```python
from build123d import *

# Parameters (mm, degrees)
EXTRUDE_1_DEPTH      = 100
SKETCH_2_R           = 40
CUT_EXTRUDE_1_DEPTH  = 90
SKETCH_9_W           = 96.5
SKETCH_9_H           = 96.5
CUT_EXTRUDE_3_DEPTH  = 100
SKETCH_15_R          = 4
EXTRUDE_4_DEPTH      = 5
SKETCH_16_R          = 29.5
CUT_EXTRUDE_5_DEPTH  = 5
SKETCH_19_W          = 96.5
SKETCH_19_H          = 96.5
CUT_EXTRUDE_8_DEPTH  = 99
SKETCH_20_R          = 2
SKETCH_20_R_2        = 4
CUT_EXTRUDE_9_DEPTH  = 1.75
SKETCH_23_W          = 92
SKETCH_23_H          = 92
EXTRUDE_5_DEPTH      = 57.3
SKETCH_24_R          = 1.75
SKETCH_24_R_2        = 4
CUT_EXTRUDE_10_DEPTH = 3
CUT_EXTRUDE_START    = -5
SKETCH_27_W          = 92
SKETCH_27_H          = 92
CUT_EXTRUDE_12_DEPTH = 50
FILLET_2_R           = 3
FILLET_6_R           = 15


with BuildPart() as part:
    # 草图1 → 凸台-拉伸1 (new body)
    with BuildSketch(Plane(origin=(0, 0, 0), x_dir=(1, 0, 0), z_dir=(0, 1, 0))):
        Polygon((-50, 50), (-50, 150), (50, 150), (150, 150), (150, 50), (50, 50), (50, -50), (-50, -50), align=None)
    extrude(amount=EXTRUDE_1_DEPTH)

    # 草图2 → 切除-拉伸1 (cut)
    with BuildSketch(Plane(origin=(0, 100, 0), x_dir=(1, 0, 0), z_dir=(0, 1, 0))):
        with Locations(Location((0, 0, 0), (0, 0, 270))):
            Circle(SKETCH_2_R)
    extrude(amount=-CUT_EXTRUDE_1_DEPTH, mode=Mode.SUBTRACT)

    # 草图9 → 切除-拉伸3 (cut)
    with BuildSketch(Plane.ZY.offset(50)):
        with Locations((0, 50)):
            Rectangle(SKETCH_9_W, SKETCH_9_H)
    extrude(amount=-CUT_EXTRUDE_3_DEPTH, mode=Mode.SUBTRACT)

    # 草图15 → 凸台-拉伸4 (add)
    with BuildSketch(Plane(origin=(0, 0, -150), x_dir=(-1, 0, 0), z_dir=(0, 0, -1))):
        with Locations(Location((-89.023351099, 21, 0), (0, 0, 180))):
            Circle(SKETCH_15_R)
        with Locations(Location((-89.023351099, 79, 0), (0, 0, 180))):
            Circle(SKETCH_15_R)
    extrude(amount=EXTRUDE_4_DEPTH)

    # 草图16 → 切除-拉伸5 (cut)
    with BuildSketch(Plane.XZ):
        with Locations((100, -100)):
            Circle(SKETCH_16_R)
    extrude(amount=-CUT_EXTRUDE_5_DEPTH, mode=Mode.SUBTRACT)

    # 草图19 → 切除-拉伸8 (cut)
    with BuildSketch(Plane.XY.offset(-50)):
        with Locations((100, 50)):
            Rectangle(SKETCH_19_W, SKETCH_19_H)
    extrude(amount=-CUT_EXTRUDE_8_DEPTH, mode=Mode.SUBTRACT)

    # 草图20 → 切除-拉伸9 (cut)
    with BuildSketch(Plane(origin=(0, 1.75, 0), x_dir=(1, 0, 0), z_dir=(0, 1, 0))):
        with Locations(Location((17.25, 0, 0), (0, 0, 270))):
            Circle(SKETCH_20_R)
        with Locations(Location((8.625, -14.938938215, 0), (0, 0, 270))):
            Circle(SKETCH_20_R)
        with Locations(Location((-8.625, -14.938938215, 0), (0, 0, 270))):
            Circle(SKETCH_20_R)
        with Locations(Location((-17.25, 0, 0), (0, 0, 270))):
            Circle(SKETCH_20_R)
        with Locations(Location((-8.625, 14.938938215, 0), (0, 0, 270))):
            Circle(SKETCH_20_R)
        with Locations(Location((8.625, 14.938938215, 0), (0, 0, 270))):
            Circle(SKETCH_20_R)
        with Locations(Location((0, 0, 0), (0, 0, 270))):
            Circle(SKETCH_20_R_2)
    extrude(amount=-CUT_EXTRUDE_9_DEPTH, mode=Mode.SUBTRACT)

    # 草图23 → 凸台-拉伸5 (add)
    with BuildSketch(Plane(origin=(0, 100, 0), x_dir=(1, 0, 0), z_dir=(0, 1, 0))):
        with Locations((100, 100)):
            Rectangle(SKETCH_23_W, SKETCH_23_H)
    extrude(amount=-EXTRUDE_5_DEPTH)

    # 草图24 → 切除-拉伸10 (cut)
    with BuildSketch(Plane.XZ.offset(-42.7)):
        with Locations(Location((100, -57.5, 0), (0, 0, 270))):
            Circle(SKETCH_24_R)
        with Locations(Location((130.0520382, -69.9479618, 0), (0, 0, 270))):
            Circle(SKETCH_24_R)
        with Locations(Location((142.5, -100, 0), (0, 0, 270))):
            Circle(SKETCH_24_R)
        with Locations(Location((130.0520382, -130.0520382, 0), (0, 0, 270))):
            Circle(SKETCH_24_R)
        with Locations(Location((100, -142.5, 0), (0, 0, 270))):
            Circle(SKETCH_24_R)
        with Locations(Location((69.9479618, -130.0520382, 0), (0, 0, 270))):
            Circle(SKETCH_24_R)
        with Locations(Location((57.5, -100, 0), (0, 0, 270))):
            Circle(SKETCH_24_R)
        with Locations(Location((69.9479618, -69.9479618, 0), (0, 0, 270))):
            Circle(SKETCH_24_R)
        with Locations(Location((100, -100, 0), (0, 0, 270))):
            Circle(SKETCH_24_R_2)
    extrude(amount=-CUT_EXTRUDE_10_DEPTH, mode=Mode.SUBTRACT)

    # 草图27 → 切除-拉伸12 (cut)
    with BuildSketch(Plane(origin=(0, 100, 0), x_dir=(1, 0, 0), z_dir=(0, 1, 0)).offset(CUT_EXTRUDE_START)):
        with Locations((98.652941691, 99.180600888)):
            Rectangle(SKETCH_27_W, SKETCH_27_H)
    extrude(amount=-CUT_EXTRUDE_12_DEPTH, mode=Mode.SUBTRACT)

    # 圆角2
    # the kernel refuses this fillet: 3 mm, written as the material it takes off along each edge
    with BuildSketch(Plane(origin=(50, -7.5, 50), x_dir=(-1, 0, 0), z_dir=(0, 1, 0)), Plane(origin=(57.5, 0, 50), x_dir=(0, 0, -1), z_dir=(-1, 0, 0)), Plane(origin=(-50, -7.5, 50), x_dir=(0, 0, -1), z_dir=(0, 1, 0)), Plane(origin=(150, 0, -157.5), x_dir=(-1, 0, 0), z_dir=(0, 0, 1))) as fillet_2_piece_1:
        with BuildLine():
            CenterArc((FILLET_2_R, -FILLET_2_R), FILLET_2_R, 90, 90)
            Line((0, -FILLET_2_R), (0, 0))
            Line((0, 0), (FILLET_2_R, 0))
        make_face()
    extrude(amount=115, mode=Mode.SUBTRACT)
    with BuildSketch(Plane(origin=(57.5, 100, 50), x_dir=(0, 0, -1), z_dir=(-1, 0, 0)), Plane(origin=(150, 100, -157.5), x_dir=(-1, 0, 0), z_dir=(0, 0, 1)), Plane(origin=(150, -7.5, -50), x_dir=(0, 0, -1), z_dir=(0, 1, 0)), Plane(origin=(150, -7.5, -150), x_dir=(-1, 0, 0), z_dir=(0, 1, 0))) as fillet_2_piece_2:
        with BuildLine():
            CenterArc((FILLET_2_R, FILLET_2_R), FILLET_2_R, 180, 90)
            Line((0, FILLET_2_R), (0, 0))
            Line((0, 0), (FILLET_2_R, 0))
        make_face()
    extrude(amount=115, mode=Mode.SUBTRACT)

    # 圆角6
    fillet_6_edges = [part.edges().sort_by_distance(p)[0] for p in [
        (-50, 50, -150),
    ]]
    fillet(fillet_6_edges, radius=FILLET_6_R)


solid = part.part
```
Check sheet for the modelled part. Datum: model origin and axes. Units: mm. A direction names the side the tool comes from. Round coordinates to 2 decimals unless told otherwise and drop trailing zeros. Write each loop counter-clockwise with the first axis right and the second up, starting at its lowest first coordinate (ties: lowest second). Pieces come first, ordered by that corner, then holes. Notation, with made-up numbers: M 88,39.5 L 96,39.5 A14 cw 96,58.5 Z; hole C 45,83.25 d11. An arc over 180 degrees is marked long. Write item = value, one per line. Start each with the question number.
1. Gauge pin test, flat ends, axial feed: pin 1 (10 mm diameter, centred on x = -22, y = 17.5, fed in from -Z); pin 2 (6.5 mm diameter, centred on x = -8.62, z = -14.94, fed in from +Y); pin 3 (16.5 mm diameter, centred on x = 99, y = 64, fed in from +Z). Record the tip position at first contact, or that the pin passes through.
2. Section check C-C, the plane x = 81.5. Record the cut outline in (y, z), then the cut area to 3 significant figures.
3. Release check for a two-part mould opening along Z. For faces 5 (the flat face through (1, 49, 50)), 6 (the flat face through (-23, 98.25, -33)), 7 (the cylindrical face through (-39.05, 99.14, -8.67)), 8 (the flat face through (-50, 49, -86)) record: pulls with the +Z half, pulls with the -Z half, needs draft (parallel to the pull), parting line crosses it, or undercut.
4. Section check D-D, the plane z = -113.5. Record the cut outline in (x, y).
5. Section check A-A, the plane x = 44.5. Record the cut outline in (y, z).
6. Tool access check on faces 1 (the flat face through (53, 98.25, -99)), 2 (the flat face through (-1, 1.75, 10)), 3 (the flat face through (51.75, 49, -99)), 4 (the cylindrical face through (127.25, 0.86, -111.3)). Record the directions out of +Z, -Z, +X, -X, +Y, -Y that give a thin tool (end or side, any length) a straight path to the whole face; none if there is none.
7. Section check B-B, the plane z = -33.5. Record the cut outline in (x, y).
8. Scan lines: line 1 (Y direction, x = 132.5, z = -139); line 2 (X direction, y = 85, z = -110); line 3 (X direction, y = 43, z = -108). Record each from-to range of solid material in increasing order. Write a range as [from, to].
Results found:
q1.pin_1 = -150
q1.pin_2 = 1.75
q1.pin_3 = -145.18
q2.outline = M 0,-150 L 100,-150 L 100,-50 L 98.25,-50 L 98.25,-54 L 95,-54 L 95,-145.18 L 45,-145.18 L 45,-54 L 42.7,-54 L 42.7,-146 L 98.25,-146 L 98.25,-149 L 1.75,-149 L 1.75,-122.98 L 0,-122.98 Z; M 0,-77.02 L 1.75,-77.02 L 1.75,-50 L 0,-50 Z
q2.area = 918 mm^2
q3.face_5 = pulls with the +Z half
q3.face_6 = undercut
q3.face_7 = undercut
q3.face_8 = needs draft
q4.outline = M -50,0 L 73.77,0 L 73.77,1.75 L 51.75,1.75 L 51.75,98.25 L 54,98.25 L 54,95 L 144.65,95 L 144.65,45 L 54,45 L 54,42.7 L 146,42.7 L 146,98.25 L 148.25,98.25 L 148.25,1.75 L 126.23,1.75 L 126.23,0 L 147,0 A3 ccw 150,3 L 150,97 A3 ccw 147,100 L -50,100 Z
q5.outline = M 0,-150 L 100,-150 L 100,47 A3 ccw 97,50 L 3,50 A3 ccw 0,47 Z; hole M 1.75,-48.25 L 98.25,-48.25 L 98.25,48.25 L 1.75,48.25 Z
q6.face_1 = none
q6.face_2 = +X, -X
q6.face_3 = +Z
q6.face_4 = -Y
q7.outline = M -50,0 L 50,0 L 50,1.75 L -50,1.75 Z; M -50,98.25 L -21.86,98.25 L -21.86,100 L -50,100 Z; M 21.86,98.25 L 50,98.25 L 50,100 L 21.86,100 Z
q8.line_1 = [0, 1.75], [42.7, 45], [95, 100]
q8.line_2 = [-50, 51.75], [144.65, 146], [148.25, 150]
q8.line_3 = [-50, 51.75], [54, 146], [148.25, 150]
